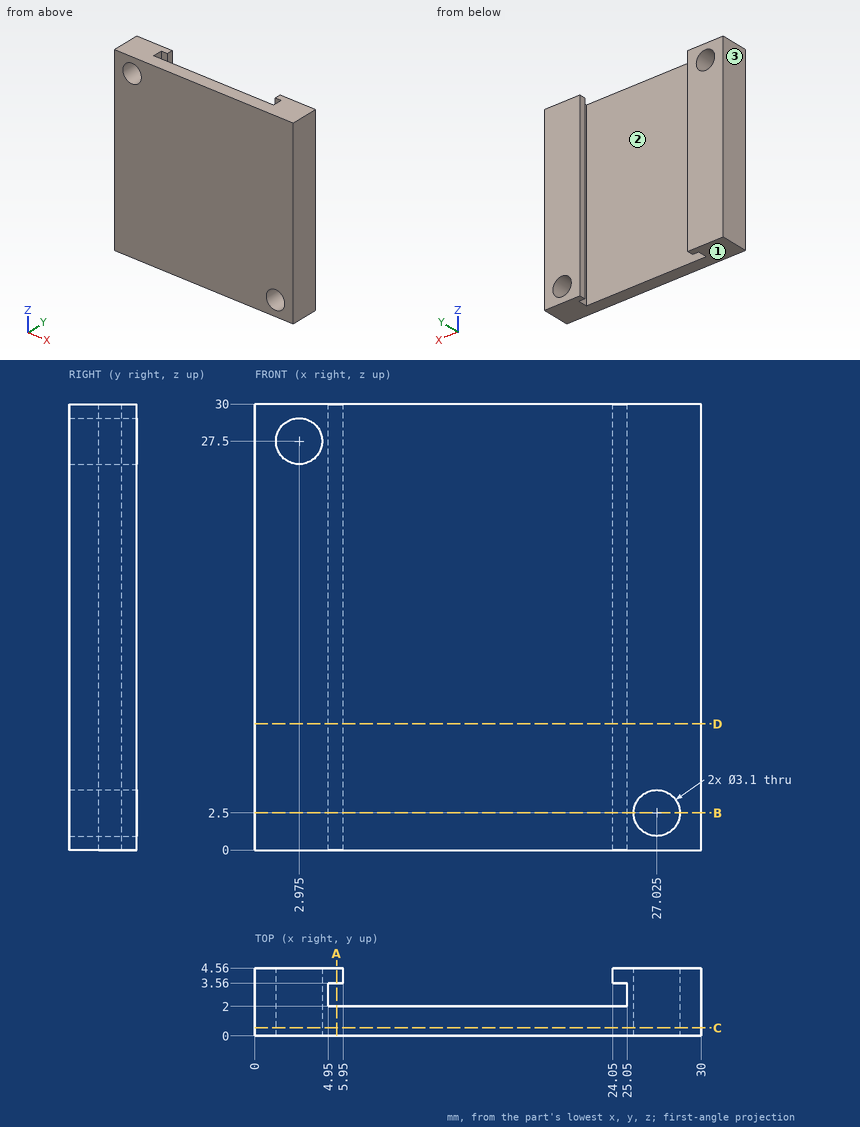
Study the drawing (mm; zero at the part's minimum x, y, z) and answer. Coordinates: 2 decimals unless noted, no trailing zeros. Order: outer loops, then holes, each group sorted by start corner. A loop starts at its lowest first (then second) coordinate and runs counter-clockwise, first axis right, second up. Notation, with made-up numbers: M -16,-38.75 L 1,-38.75 A24 cw 1,-7.75 Z; hole C -3.75,-20.5 d6. An arc over 180 degrees is marked long. Answer as a JSON object with one key per item and string values. Group by question number.
1. Flat-ended cylindrical pins translate along their axes: P1, Ø2.5, axis at x = 2.975, z = 27.5, coming from the -Y side; P2, Ø1.5, axis at x = 14.5, z = 25.5, coming from the +Y side. Find the tip coordinate at first contact, or state that the pin passes through.
2. Determine the mould class of the marked faces 1, 2 and 3 for opening direction X: released by +X, released by -X, zero draft, split by the parting line, or undercut.
3. Section B-B on z = 2.5 is taken. Write down the section's boundary in (x, y) (3 decimals), then the cut area to 3 significant figures.
4. Section C-C on y = 0.55 is taken. Write down the section's boundary in (x, z) (3 decimals), then the cut area to 3 significant figures.
5. Straight lines are drawn through the part: line 1 (X direction, y = 2.7, z = 27.5) (3 decimals); line 2 (X direction, y = 1.65, z = 27.5) (3 decimals); line 3 (X direction, y = 2.7, z = 7.25). For each, find the intervals that lie inside material, in ascending order.
6. Section D-D on z = 8.5 is taken. Write down the section's boundary in (x, y), then the cut area to 3 significant figures.
7. Section A-A on x = 5.5 is taken. Write down the section's boundary in (y, z), then the cut area to 3 significant figures.
Values follow:
{
 "1": {"P1": "through", "P2": "y = 2"},
 "2": {"face 1": "zero draft", "face 2": "undercut", "face 3": "released by -X"},
 "3": {"outline": "M 0,0 L 25.475,0 L 25.475,4.56 L 24.05,4.56 L 24.05,3.56 L 25.05,3.56 L 25.05,2 L 4.95,2 L 4.95,3.56 L 5.95,3.56 L 5.95,4.56 L 0,4.56 Z; M 28.575,0 L 30,0 L 30,4.56 L 28.575,4.56 Z", "area": "73.2 mm2"},
 "4": {"outline": "M 0,0 L 30,0 L 30,30 L 0,30 Z; hole C 2.975,27.5 d3.1; hole C 27.025,2.5 d3.1", "area": "885 mm2"},
 "5": {"line 1": "0 to 1.425, 4.525 to 4.95, 25.05 to 30", "line 2": "0 to 1.425, 4.525 to 30", "line 3": "0 to 4.95, 25.05 to 30"},
 "6": {"outline": "M 0,0 L 30,0 L 30,4.56 L 24.05,4.56 L 24.05,3.56 L 25.05,3.56 L 25.05,2 L 4.95,2 L 4.95,3.56 L 5.95,3.56 L 5.95,4.56 L 0,4.56 Z", "area": "87.3 mm2"},
 "7": {"outline": "M 0,0 L 2,0 L 2,30 L 0,30 Z; M 3.56,0 L 4.56,0 L 4.56,30 L 3.56,30 Z", "area": "90.0 mm2"}
}
